Work out the finished part from the listing and answer in its coordinate system (mm). Face numbers are marked on the shaded views. A direction names the side the tool comes from. Give positions to 0.01 mm unless a question says otherwise; leave off trailing zeros. Loops run counter-clockwise (first coordinate to the right, second up) from the corner with the lowest first, then second, coordinate; pieces in that order, holes last. Notation, with made-up numbers: (13.25, -31.75) -> (64.25, -31.75) arc R31 ccw to (64.25, 1.25) -> close; hole circle Ø10 at (69.25, 26.25). An arc over 180 degrees is marked (long way). Answer as CSV lines item,"result". Start each with the question number.
1. Find the intervals of material crossed by line 1 along Y through (x, z) = (-1.5, 0) (3 decimals); line 2 along Y through (x, z) = (-3, 0); line 3 along Z through (x, y) = (-4.75, 9.5), in increasing order.
2. A tool of negligible diameter and unlimited length cuts with its end or side. For the marked faces 3 and 4, from which of +Z, -Z, +X, -X, +Y, -Y can it reach the whole face along a straight path? Write none if from no direction.
3. Find section B-B, the plane x = -28.5. Give the vertices of the cut face in (y, z).
4. Flat-ended cylindrical pins translate along their axes: pin 1 Ø1 at (x, z) = (8.5, -1) entering from -Y; pin 2 Ø1 at (x, z) = (-7, -5) entering from -Y; pin 3 Ø10 at (y, z) = (11.5, 7) entering from -X. Find the tip coordinate at first contact, or state that the pin passes through.
5. Find section A-A, the plane x = 11. Give the vertices of the cut face in (y, z).
6. Determine the mould class of the marked faces 1 and 2 for opening direction Z: +Z half, -Z half, draft (parallel to the pull), parting line (faces both ways), or undercut.
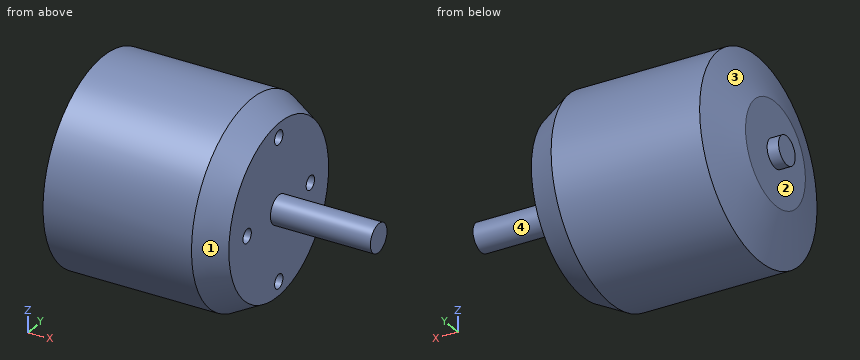
from build123d import *

# Parameters (mm, degrees)
SKETCH1_3_W               = 17.5
SKETCH1_3_H               = 2.5
SKETCH1_3_W_2             = 2
M3X0_5_TAPPED_HOLE1_D     = 2.5
M3X0_5_TAPPED_HOLE1_DEPTH = 7.5
M3X0_5_TAPPED_HOLE1_TIP   = 0.751075774


with BuildPart() as part:
    # Sketch1 → Revolve1 (revolve)
    with BuildSketch(Plane.XY, mode=Mode.PRIVATE) as revolve1_sk:
        Polygon((0, 0), (-34, 0), (-34, 2.5), (-34, 9), (-31, 17.65), (-5, 17.65), (0, 15), (0, 2.5), align=None)
    revolve(revolve1_sk.sketch.rotate(Axis((1.227272727, 0, 0), (1, 0, 0)), 90), axis=Axis((1.227272727, 0, 0), (1, 0, 0)))

    # Sketch1_3 → Revolve2 (revolve)
    with BuildSketch(Plane.XY, mode=Mode.PRIVATE) as revolve2_sk:
        with Locations((8.75, 1.25)):
            Rectangle(SKETCH1_3_W, SKETCH1_3_H)
        with Locations((-35, 1.25)):
            Rectangle(SKETCH1_3_W_2, SKETCH1_3_H)
    revolve(revolve2_sk.sketch.rotate(Axis((1.227272727, 0, 0), (1, 0, 0)), 90), axis=Axis((1.227272727, 0, 0), (1, 0, 0)))

    # M3x0.5 Tapped Hole1
    with Locations(Plane(origin=(0, 0, 0), x_dir=(0, 0, -1), z_dir=(1, 0, 0))):
        with Locations((0, 9.5), (0, -9.5), (-12.5, 0), (12.5, 0)):
            Hole(M3X0_5_TAPPED_HOLE1_D / 2, depth=M3X0_5_TAPPED_HOLE1_DEPTH)
            with Locations((0, 0, -(M3X0_5_TAPPED_HOLE1_DEPTH + M3X0_5_TAPPED_HOLE1_TIP / 2))):  # 118° drill point
                Cone(0, M3X0_5_TAPPED_HOLE1_D / 2, M3X0_5_TAPPED_HOLE1_TIP, mode=Mode.SUBTRACT)


solid = part.part
Resolved:
1,line 1,"y = -15.795 to -10.75, -8.25 to 8.25, 10.75 to 15.795"
1,line 2,"y = -16.59 to -10.75, -8.25 to 8.25, 10.75 to 16.59"
1,line 3,"z = -14.72 to -1.25, 1.25 to 14.72"
2,face 3,"-X"
2,face 4,"+X"
3,outline,"circle Ø35.3 at (0, 0)"
4,pin 1,"stops at y = -2.45"
4,pin 2,"stops at y = -17.07"
4,pin 3,"stops at x = -34"
5,outline,"circle Ø5 at (0, 0)"
6,face 1,"parting line"
6,face 2,"draft"
